```python
from build123d import *

# Parameters (mm, degrees)
ESQUISSE4_W             = 400
ESQUISSE4_H             = 300
BOSS_EXTRU_1_DEPTH      = 325.81
ENL_V_MAT_EXTRU_1_DEPTH = 597.784849087
ENL_V_MAT_EXTRU_3_DEPTH = 758.184749953


with BuildPart() as part:
    # Esquisse4 → Boss.-Extru.1 (new body)
    with BuildSketch(Plane.XY):
        with Locations((200, 237.392658036)):
            Rectangle(ESQUISSE4_W, ESQUISSE4_H)
    extrude(amount=-BOSS_EXTRU_1_DEPTH)

    # Esquisse9 → Enlèv. mat.-Extru.1 (cut, through all)
    with BuildSketch(Plane(origin=(0, 387.392658036, 0), x_dir=(1, 0, 0), z_dir=(0, 1, 0))):
        Polygon((0, 0), (200, 325.81), (400, 0), (400, 335.81), (0, 335.81), align=None)
    extrude(amount=-ENL_V_MAT_EXTRU_1_DEPTH, mode=Mode.SUBTRACT)

    # Esquisse10 → Enlèv. mat.-Extru.3 (cut, through all, along a direction that is not the sketch's normal)
    with BuildSketch(Plane(origin=(0, 0, 0), x_dir=(-0.5231513885267656, 0, 0.8522397694795271), z_dir=(-0.8522397694795271, 0, -0.5231513885267656))):
        Polygon((0, 387.392658036), (-382.298516999, 237.392658036), (0, 87.392658036), (-392.298516999, 87.392658036), (-392.298516999, 387.392658036), align=None)
    extrude(amount=-ENL_V_MAT_EXTRU_3_DEPTH, dir=(-1, 0, 0), mode=Mode.SUBTRACT)


solid = part.part
```
Could you check a few things on this model? Use its own coordinates, in mm. Give positions to 0.01 mm unless a question says otherwise; leave off trailing zeros. Loops run counter-clockwise (first coordinate to the right, second up) from the corner with the lowest first, then second, coordinate; pieces in that order, holes last. Notation, with made-up numbers: (-38.75, -1) - (-30.75, -1) arc R11 cw to (-30.75, 20) - close; hole circle Ø5 at (-20, 86). An arc over 180 degrees is marked (long way). Answer in a Markdown table with one row per item. Add a question column.
Q1. For pin 1 (6 mm diameter, centred on y = 282, z = -63.5, fed in from -X); pin 2 (5 mm diameter, centred on x = 124.5, y = 245.5, fed in from -Z); pin 3 (1.5 mm diameter, centred on x = 287.5, y = 129.5, fed in from -Z), each with a flat end and sliding along its axis, tell me the tip position at first contact or that it passes through.
Q2. If we section it at B-B (x = 40.5): List the corners of the cut face in (y, z) for me, plus the area to 3 significant figures.
Q3. If we section it at A-A (y = 145): List the corners of the cut face in (x, z) for me, plus the area to 3 significant figures.
Q4. Please list where these lines run through material, in increasing order: L1, parallel to Y at x = 145, z = -184; L2, parallel to Z at x = 311, y = 230.5; L3, parallel to Z at x = 170.5, y = 267. Write a range as from..to.
The answers:
| question | item | result |
|---|---|---|
| 1 | pin 1 | stops at x = 37.14 |
| 1 | pin 2 | stops at z = -206.89 |
| 1 | pin 3 | stops at z = -93.09 |
| 2 | outline | (87.39, 0) - (117.77, -65.98) - (357.02, -65.98) - (387.39, 0) - close |
| 2 | area | 17,800 mm^2 |
| 3 | outline | (0, 0) - (76.81, -125.13) - (323.19, -125.13) - (400, 0) - close |
| 3 | area | 40,400 mm^2 |
| 4 | L1 | y = 172.1..302.68 |
| 4 | L2 | z = -144.99..0 |
| 4 | L3 | z = -261.5..0 |
